Part model, mm, in its own coordinate system. A direction names the side the tool comes from. Round coordinates to 2 decimals unless told otherwise and drop trailing zeros. Loops run counter-clockwise (first coordinate to the right, second up) from the corner with the lowest first, then second, coordinate; pieces in that order, holes last. Notation, with made-up numbers: M 76.25,-31.5 L 104.25,-31.5 A7 cw 104.25,-23.5 Z; hole C 30,81 d9. An arc over 180 degrees is marked long. Put each result on its own line as item: value. Start each with the question number.
1) Slice it at D-D on x = -1. Give the cut face in (y, z), then the cut area to 3 significant figures.
2) Drop flat-ended pins along their axis: pin 1 Ø1 at (x, y) = (3, 8.5) entering from +Z; pin 2 Ø3 at (x, y) = (2.5, 12) entering from -Z; pin 3 Ø2.5 at (x, z) = (0, 0) entering from +Y. Give the stop position or say it passes through.
3) Probe line 1 along Y through (x, z) = (0, 2.85); line 2 along Y through (x, z) = (0, -1); line 3 along X through (y, z) = (4.25, 1.5). List the from-to ranges inside material, lowest first.
4) Slice it at A-A on x = 0. Give the cut face in (y, z).
5) Slice it at C-C on y = 6.75. Give the cut face in (x, z), then the cut area to 3 significant figures.
6) Slice it at B-B on z = 0. Give the cut face in (x, y).
7) Which spindle directions (+Z, -Z, +X, -X, +Y, -Y) get a long thin tool onto all of the face, cutting with end or side? Do faces 4 (the cylindrical face through (0.8, 5, 2.9)), 5 (the cylindrical face through (0.766, 5.169, -1.847)), 6 (the cylindrical face through (-1, 18.07, -1.31)). Say none if no direction does.
8) Pull direction X, two halves, no side cores. Call faces 1 (the flat face through (-1, 3, 2)), 2 (the cylindrical face through (-3.905, 12.86, -0.867)), 3 (the flat face through (0, 13, 0)): +X half, -X half, draft (parallel to the pull), parting line (faces both ways), or undercut.
```python
from build123d import *

# Parameters (mm, degrees)
CROQUIS1_R              = 4
CROQUIS1_R_2            = 2
SALIENTE_EXTRUIR1_DEPTH = 25.4
CROQUIS2_R              = 30
SALIENTE_EXTRUIR2_DEPTH = 5
CROQUIS3_R              = 2
CORTAR_EXTRUIR1_DEPTH   = 7.5
CROQUIS7_R              = 3.5
CORTAR_EXTRUIR3_DEPTH   = 3
CROQUIS8_W              = 62.698346187
CROQUIS8_H              = 3
CORTAR_EXTRUIR5_DEPTH   = 15
CROQUIS1_3_R            = 2
CORTAR_EXTRUIR6_DEPTH   = 7.4
CROQUIS6_R              = 0.8
CORTAR_EXTRUIR7_DEPTH   = 10
CROQUIS10_R             = 30
CORTAR_EXTRUIR8_DEPTH   = 7.4
CROQUIS11_R             = 1.65
CORTAR_EXTRUIR9_DEPTH   = 10


with BuildPart() as part:
    # Croquis1 → Saliente-Extruir1 (new body)
    with BuildSketch(Plane(origin=(0, 0, 0), x_dir=(1, 0, 0), z_dir=(0, 1, 0))):
        with Locations(Location((0, 0, 0), (0, 0, 270))):
            Circle(CROQUIS1_R)
        Circle(CROQUIS1_R_2, mode=Mode.SUBTRACT)
        Circle(CROQUIS1_R_2)
    extrude(amount=SALIENTE_EXTRUIR1_DEPTH)

    # Croquis2 → Saliente-Extruir2 (add)
    with BuildSketch(Plane(origin=(0, 25.4, 0), x_dir=(1, 0, 0), z_dir=(0, 1, 0))):
        with Locations(Location((0, 0, 0), (0, 0, 270))):
            Circle(CROQUIS2_R)
    extrude(amount=SALIENTE_EXTRUIR2_DEPTH)

    # Croquis3 → Cortar-Extruir1 (cut)
    with BuildSketch(Plane(origin=(0, 30.4, 0), x_dir=(1, 0, 0), z_dir=(0, 1, 0))):
        with Locations(Location((0, 10, 0), (0, 0, 270))):
            Circle(CROQUIS3_R)
        with Locations(Location((10, 0, 0), (0, 0, 270))):
            Circle(CROQUIS3_R)
        with Locations(Location((0, -10, 0), (0, 0, 270))):
            Circle(CROQUIS3_R)
        with Locations(Location((-10, 0, 0), (0, 0, 270))):
            Circle(CROQUIS3_R)
    extrude(amount=-CORTAR_EXTRUIR1_DEPTH, mode=Mode.SUBTRACT)

    # Croquis7 → Cortar-Extruir3 (cut)
    with BuildSketch(Plane.XZ):
        with Locations(Location((0, 0, 0), (0, 0, 270))):
            Circle(CROQUIS7_R)
    extrude(amount=-CORTAR_EXTRUIR3_DEPTH, mode=Mode.SUBTRACT)

    # Croquis8 → Cortar-Extruir5 (cut, symmetric)
    with BuildSketch(Plane(origin=(0, 0, 0), x_dir=(0, 0, -1), z_dir=(1, 0, 0))):
        with Locations((4.276742622, 1.5)):
            Rectangle(CROQUIS8_W, CROQUIS8_H)
    extrude(amount=CORTAR_EXTRUIR5_DEPTH, both=True, mode=Mode.SUBTRACT)

    # Croquis1<3> → Cortar-Extruir6 (cut)
    with BuildSketch(Plane(origin=(0, 0, 0), x_dir=(1, 0, 0), z_dir=(0, 1, 0))):
        with Locations(Location((0, 0, 0), (0, 0, 90))):
            Circle(CROQUIS1_3_R)
    extrude(amount=CORTAR_EXTRUIR6_DEPTH, mode=Mode.SUBTRACT)

    # Croquis6 → Cortar-Extruir7 (cut)
    with BuildSketch(Plane.XY):
        with Locations(Location((0, 5, 0), (0, 0, 180))):
            Circle(CROQUIS6_R)
    extrude(amount=CORTAR_EXTRUIR7_DEPTH, mode=Mode.SUBTRACT)

    # Croquis10 → Cortar-Extruir8 (cut)
    with BuildSketch(Plane(origin=(0, 30.4, 0), x_dir=(1, 0, 0), z_dir=(0, 1, 0))):
        Circle(CROQUIS10_R)
    extrude(amount=-CORTAR_EXTRUIR8_DEPTH, mode=Mode.SUBTRACT)

    # Croquis11 → Cortar-Extruir9 (cut)
    with BuildSketch(Plane(origin=(0, 23, 0), x_dir=(1, 0, 0), z_dir=(0, 1, 0))):
        with Locations(Location((0, 0, 0), (0, 0, 270))):
            Circle(CROQUIS11_R)
    extrude(amount=-CORTAR_EXTRUIR9_DEPTH, mode=Mode.SUBTRACT)


solid = part.part
```
Recorded:
1. outline: M 3,-3.87 L 23,-3.87 L 23,-1.31 L 13,-1.31 L 13,1.31 L 23,1.31 L 23,3.87 L 3,3.87 L 3,1.73 L 7.4,1.73 L 7.4,-1.73 L 3,-1.73 Z
1. area: 113 mm2
2. pin 1: stops at z = 3.12
2. pin 2: stops at z = -3.87
2. pin 3: stops at y = 13
3. line 1: y = 3 to 4.2, 5.8 to 23
3. line 2: y = 7.4 to 13
3. line 3: x = -3.71 to -1.32, 1.32 to 3.71
4. outline: M 3,-4 L 23,-4 L 23,-1.65 L 13,-1.65 L 13,1.65 L 23,1.65 L 23,4 L 5.8,4 L 5.8,2 L 7.4,2 L 7.4,-2 L 3,-2 Z; M 3,2 L 4.2,2 L 4.2,4 L 3,4 Z
5. outline: C 0,0 d8; hole C 0,0 d4
5. area: 37.7 mm2
6. outline: M -4,3 L -2,3 L -2,7.4 L 2,7.4 L 2,3 L 4,3 L 4,23 L 1.65,23 L 1.65,13 L -1.65,13 L -1.65,23 L -4,23 Z
7. face 4: +Z
7. face 5: -Y
7. face 6: +Y
8. face 1: draft
8. face 2: parting line
8. face 3: undercut
